```python
from build123d import *

# Parameters (mm, degrees)
F0_R     = 3.175
F1_DEPTH = 6.35
F3_DEPTH = 127


with BuildPart() as f1:
    # F0 (on Top) → F1 (new body, symmetric)
    with BuildSketch(Plane.XY):
        Polygon((0, -6.35), (0, 0), (0, 6.35), (-12.7, 6.35), (-76.2, 6.35), (-76.2, -6.35), align=None)
        with Locations((-63.5, 0)):
            Circle(F0_R, mode=Mode.SUBTRACT)
        with BuildLine():
            ThreePointArc((-9.525, 0), (-14.945064, -2.245064), (-12.7, 3.175))
            ThreePointArc((-12.7, 3.175), (-10.454936, 2.245064), (-9.525, 0))
        make_face(mode=Mode.SUBTRACT)
    extrude(amount=F1_DEPTH, both=True)

    # F2 (on face) → F3 (join)
    with BuildSketch(Plane.YZ):
        with BuildLine():
            ThreePointArc((0, -6.35), (4.490128, -4.490128), (6.35, 0))
            ThreePointArc((6.35, 0), (4.490128, 4.490128), (0, 6.35))
            ThreePointArc((0, 6.35), (-4.490128, 4.490128), (-6.35, 0))
            ThreePointArc((-6.35, 0), (-4.490128, -4.490128), (0, -6.35))
        make_face()
    extrude(amount=F3_DEPTH)


solid = f1.part
```
CAD build for the part. Positions are in the model's coordinates, mm. A direction names the side the tool comes from. Round coordinates to 2 decimals unless told otherwise and drop trailing zeros. Order: outer loops, then holes, each group sorted by start corner. A loop starts at its lowest first (then second) coordinate and runs counter-clockwise, first axis right, second up. Notation, with made-up numbers: (12.25, -39.75) -> (57.25, -39.75) arc R17 cw to (57.25, -9.75) -> close; hole circle Ø5 at (42.5, 38.25). An arc over 180 degrees is marked (long way). One line per question, with ' | ' between items.
Q1. Probe probe 1 along Y at (x, z) = (-63.5, 1.25) (3 decimals); probe 2 along Z at (x, y) = (31, 0.5). List the from-to ranges inside material, lowest first.
Completed:
probe 1: y = -6.35 to -3.175, 3.175 to 6.35 | probe 2: z = -6.33 to 6.33
Q2. Which spindle directions (+Z, -Z, +X, -X, +Y, -Y) get a long thin tool onto all of the face, cutting with end or side? Do faces 4 (the flat face through (0, 5, -5)), 5 (the flat face through (0, 5, 5)), 6 (the flat face through (0, -5, -5)). Say none if no direction does.
Completed:
face 4: -Z, +X, +Y | face 5: +Z, +X, +Y | face 6: -Z, +X, -Y
Q3. Two-plate mould, pull along Y, no slides. Class faces 1 (the flat face through (-76.2, 0, 0)), 2 (the cylindrical face through (-60.47, 0.95, -0.09)), 3 (the flat face through (-39, -6.35, 0)): released by +Y, released by -Y, zero draft, split by the parting line, or undercut.
Completed:
face 1: zero draft | face 2: undercut | face 3: released by -Y
Q4. Slice it at A-A (x = -63.5). Write the cut outline in (y, z) (3 decimals).
Completed:
outline: (-6.35, -6.35) -> (-3.175, -6.35) -> (-3.175, 6.35) -> (-6.35, 6.35) -> close; (3.175, -6.35) -> (6.35, -6.35) -> (6.35, 6.35) -> (3.175, 6.35) -> close
Q5. Drop a flat-ended pin along its axis: pin 1 (3 mm diameter, centred on x = 49, y = -1.5, fed in from -Z). Give the stop position or say it passes through.
Completed:
pin 1: stops at z = -6.35
Q6. Slice it at C-C (x = 13). Write the cut outline in (y, z), then the cut area to 3 significant figures.
Completed:
outline: circle Ø12.7 at (0, 0) | area: 127 mm^2
Q7. Slice it at B-B (z = -2.75). Write the cut outline in (x, y) (3 decimals), then the cut area to 3 significant figures.
Completed:
outline: (-76.2, -6.35) -> (0, -6.35) -> (0, -5.724) -> (127, -5.724) -> (127, 5.724) -> (0, 5.724) -> (0, 6.35) -> (-76.2, 6.35) -> close; hole circle Ø6.35 at (-63.5, 0); hole circle Ø6.35 at (-12.7, 0) | area: 2,360 mm^2
